from build123d import *

# Parameters (mm, degrees)
CROQUIS1_W              = 340
CROQUIS1_H              = 260
SALIENTE_EXTRUIR1_DEPTH = 270
CROQUIS2_W              = 334
CROQUIS2_H              = 254
CORTAR_EXTRUIR1_DEPTH   = 267
CORTAR_EXTRUIR2_DEPTH   = 341


with BuildPart() as part:
    # Croquis1 → Saliente-Extruir1 (new body)
    with BuildSketch(Plane(origin=(0, 0, 0), x_dir=(1, 0, 0), z_dir=(0, 1, 0))):
        Rectangle(CROQUIS1_W, CROQUIS1_H)
    extrude(amount=SALIENTE_EXTRUIR1_DEPTH)

    # Croquis2 → Cortar-Extruir1 (cut)
    with BuildSketch(Plane.XZ):
        Rectangle(CROQUIS2_W, CROQUIS2_H)
    extrude(amount=-CORTAR_EXTRUIR1_DEPTH, mode=Mode.SUBTRACT)

    # Croquis3 → Cortar-Extruir2 (cut, through all)
    with BuildSketch(Plane(origin=(170, 0, 0), x_dir=(0, 0, -1), z_dir=(1, 0, 0))):
        Polygon((0, 0), (-82, 0), (-82, 30), (-30, 30), (-30, 55), (30, 55), (30, 30), (82, 30), (82, 0), align=None)
    extrude(amount=-CORTAR_EXTRUIR2_DEPTH, mode=Mode.SUBTRACT)


solid = part.part
Could you check a few things on this model? Use its own coordinates, in mm. A direction names the side the tool comes from. Give positions to 0.01 mm unless a question says otherwise; leave off trailing zeros. Loops run counter-clockwise (first coordinate to the right, second up) from the corner with the lowest first, then second, coordinate; pieces in that order, holes last. Notation, with made-up numbers: (81.25, 88) -> (127.25, 88) arc R17 ccw to (127.25, 109) -> close; hole circle Ø1 at (79.5, 64.25). An arc over 180 degrees is marked (long way). Answer as CSV lines item,"result". Start each with the question number.
(1) Which directions (+Z, -Z, +X, -X, +Y, -Y) give clear straight access to the entire face, cutting with the end or side of a thin tool? Please do faces 1 (the flat face through (-1, 0, -129)), 2 (the flat face through (-2, 132, 127)).
(2) If we section it at A-A on y = 196: Write out the boundary of the cut face in (x, z).
(3) If we section it at D-D on x = -41.5: Write out the boundary of the cut face in (y, z).
(4) We'd pull the mould along Z, two halves only. Please class faces 3 (the flat face through (170, 133, 2)), 4 (the flat face through (-2, 133, -130)), 5 (the flat face through (-2, 132, -127)): released by +Z, released by -Z, zero draft, split by the parting line, or undercut.
(5) I need wall thicknesses on probe 1 along X at (y, z) = (163, -88); probe 2 along Z at (x, y) = (-106, 192.5); probe 3 along Y at (x, z) = (-6.5, 111). Which ranges of each line are inside material? Lowest first, please.
(6) If we section it at B-B on y = 21: Write out the boundary of the cut face in (x, z), then the cut area to 3 significant figures.
(7) I'm going to push flat-ended pins straight in: pin 1 Ø1.5 at (x, z) = (-169, -63) entering from -Y; pin 2 Ø10 at (x, z) = (-31.5, -26.5) entering from -Y; pin 3 Ø1.5 at (x, z) = (168, -2.5) entering from -Y. Where does each tip first touch, or does it pass through?
(8) If we section it at C-C on z = 4: Write out the boundary of the cut face in (x, y).
Computed:
1,face 1,"+Z, -Z, +X, -X, -Y"
1,face 2,"-Y"
2,outline,"(-170, -130) -> (170, -130) -> (170, 130) -> (-170, 130) -> close; hole (-167, -127) -> (167, -127) -> (167, 127) -> (-167, 127) -> close"
3,outline,"(0, -130) -> (270, -130) -> (270, 130) -> (0, 130) -> (0, 127) -> (267, 127) -> (267, -127) -> (0, -127) -> close"
4,face 3,"zero draft"
4,face 4,"released by -Z"
4,face 5,"undercut"
5,probe 1,"x = -170 to -167, 167 to 170"
5,probe 2,"z = -130 to -127, 127 to 130"
5,probe 3,"y = 267 to 270"
6,outline,"(-170, -130) -> (170, -130) -> (170, -82) -> (167, -82) -> (167, -127) -> (-167, -127) -> (-167, -82) -> (-170, -82) -> close; (-170, 82) -> (-167, 82) -> (-167, 127) -> (167, 127) -> (167, 82) -> (170, 82) -> (170, 130) -> (-170, 130) -> close"
6,area,"2,580 mm2"
7,pin 1,"stops at y = 30"
7,pin 2,"stops at y = 267"
7,pin 3,"stops at y = 55"
8,outline,"(-170, 55) -> (-167, 55) -> (-167, 267) -> (167, 267) -> (167, 55) -> (170, 55) -> (170, 270) -> (-170, 270) -> close"
